CAD build for the part. Positions are in the model's coordinates, mm. A direction names the side the tool comes from. Round coordinates to 2 decimals unless told otherwise and drop trailing zeros. Loops run counter-clockwise (first coordinate to the right, second up) from the corner with the lowest first, then second, coordinate; pieces in that order, holes last.
```python
from build123d import *

# Parameters (mm, degrees)
F0_R     = 13.97
F1_DEPTH = 15.875
F2_R     = 5.08
F3_SIZE2 = 1.27
F3_SIZE  = 1.27
F4_R     = 3.683
F5_DEPTH = 1.778
F6_R     = 1.905
F7_DEPTH = 7.621


with BuildPart() as f1:
    # F0 (on Top) → F1 (new body, symmetric)
    with BuildSketch(Plane.XY):
        with BuildLine():
            Line((3.81, 38.1), (-3.81, 38.1))
            Line((-3.81, 38.1), (-3.81, 23.11151))
            Line((-3.81, 23.11151), (-19.05, 12.95151))
            ThreePointArc((-19.05, 12.95151), (-52.07, 0), (-19.05, -12.95151))
            Line((-19.05, -12.95151), (-3.81, -23.11151))
            Line((-3.81, -23.11151), (-3.81, -38.1))
            Line((-3.81, -38.1), (3.81, -38.1))
            Line((3.81, -38.1), (3.81, 38.1))
        make_face()
        with Locations((-33.02, 0)):
            Circle(F0_R, mode=Mode.SUBTRACT)
    extrude(amount=F1_DEPTH, both=True)

    # F2
    f2_edges = [f1.edges().sort_by_distance(p)[0] for p in [
        (-19.05, -12.95151, 0),
        (-3.81, -23.11151, 0),
        (-3.81, 23.11151, 0),
        (-19.05, 12.95151, 0),
    ]]
    fillet(f2_edges, radius=F2_R)

    # F3
    f3_edges = [f1.edges().sort_by_distance(p)[0] for p in [
        (-46.99, 0, 15.875),
        (-46.99, 0, -15.875),
    ]]
    chamfer(f3_edges, length=F3_SIZE, length2=F3_SIZE2)

    # F4 (on face) → F5 (cut)
    with BuildSketch(Plane(origin=(-3.81, 0, 0), x_dir=(0, -1, 0), z_dir=(-1, 0, 0))):
        with Locations((-31.75, 8.255)):
            Circle(F4_R)
        with Locations((-31.75, -8.255)):
            Circle(F4_R)
        with Locations((31.75, 8.255)):
            Circle(F4_R)
        with Locations((31.75, -8.255)):
            Circle(F4_R)
    extrude(amount=-F5_DEPTH, mode=Mode.SUBTRACT)

    # F6 (on face) → F7 (cut, through all)
    with BuildSketch(Plane(origin=(-3.81, 0, 0), x_dir=(0, -1, 0), z_dir=(-1, 0, 0))):
        with Locations((31.75, 8.255)):
            Circle(F6_R)
        with Locations((-31.75, 8.255)):
            Circle(F6_R)
        with Locations((31.75, -8.255)):
            Circle(F6_R)
        with Locations((-31.75, -8.255)):
            Circle(F6_R)
    extrude(amount=-F7_DEPTH, mode=Mode.SUBTRACT)


solid = f1.part
```
Item 1: Cut at A-A, the plane y = 31.75. Give the cut face in (x, z) (3 decimals), plus the area to 3 significant figures.
Answers follow:
outline: (-3.81, -15.875) - (3.81, -15.875) - (3.81, -10.16) - (-2.032, -10.16) - (-2.032, -11.938) - (-3.81, -11.938) - close; (-3.81, -4.572) - (-2.032, -4.572) - (-2.032, -6.35) - (3.81, -6.35) - (3.81, 6.35) - (-2.032, 6.35) - (-2.032, 4.572) - (-3.81, 4.572) - close; (-3.81, 11.938) - (-2.032, 11.938) - (-2.032, 10.16) - (3.81, 10.16) - (3.81, 15.875) - (-3.81, 15.875) - close
area: 171 mm2
Item 2: Cut at C-C, the plane x = -33.02. Give the cut face in (y, z) (3 decimals), plus the area to 3 significant figures.
Answers follow:
outline: (-19.05, -15.875) - (-15.24, -15.875) - (-13.97, -14.605) - (-13.97, 14.605) - (-15.24, 15.875) - (-19.05, 15.875) - close; (13.97, -14.605) - (15.24, -15.875) - (19.05, -15.875) - (19.05, 15.875) - (15.24, 15.875) - (13.97, 14.605) - close
area: 319 mm2
Item 3: Cut at D-D, the plane y = 0. Give the cut face in (x, z) (3 decimals), plus the area to 3 significant figures.
Answers follow:
outline: (-52.07, -15.875) - (-48.26, -15.875) - (-46.99, -14.605) - (-46.99, 14.605) - (-48.26, 15.875) - (-52.07, 15.875) - close; (-19.05, -14.605) - (-17.78, -15.875) - (3.81, -15.875) - (3.81, 15.875) - (-17.78, 15.875) - (-19.05, 14.605) - close
area: 884 mm2
Item 4: Cut at B-B, the plane z = 0.5. Give the cut face in (x, y), plus the area to 3 significant figures.
Answers follow:
outline: (-21.64, -15.28) arc R5.08 cw to (-15.79, -15.13) - (-6.07, -21.6) arc R5.08 cw to (-3.81, -25.83) - (-3.81, -38.1) - (3.81, -38.1) - (3.81, 38.1) - (-3.81, 38.1) - (-3.81, 25.83) arc R5.08 cw to (-6.07, 21.6) - (-15.79, 15.13) arc R5.08 cw to (-21.64, 15.28) arc R19.05 ccw (long way) to start; hole circle Ø27.94 at (-33.02, 0)
area: 1,570 mm2
Item 5: 3-axis set-ups, long thin cutter, end or side, ignore diameter. For faces 1 (the flat face through (-12, 0, 15.875)), 2 (the cylindrical face through (-2.933, 34.465, 10.744)), 3 (the flat face through (-3.81, -32, 0)): which of +Z, -Z, +X, -X, +Y, -Y reach the whole face in a straight line?
Answers follow:
face 1: +Z, +X, -X, +Y, -Y
face 2: -X
face 3: +Z, -Z, -X, -Y
Item 6: Two-plate mould, pull along X, no slides. Class faces 4 (the flat face through (-3.81, 32, 0)), 5 (the cylindrical face through (0.848, -29.847, -8.171)), 6 (the cylindrical face through (-52.06, 0.59, 0.22)): released by +X, released by -X, zero draft, split by the parting line, or undercut.
Answers follow:
face 4: released by -X
face 5: zero draft
face 6: undercut
Item 7: Probe line 1 (Z direction, x = -2.65, y = 31.75) (3 decimals); line 2 (Z direction, x = 1, y = 31) (3 decimals); line 3 (Y direction, x = -39, z = -7). List the from-to ranges inside material, lowest first.
Answers follow:
line 1: z = -15.875 to -11.938, -4.572 to 4.572, 11.938 to 15.875
line 2: z = -15.875 to -10.006, -6.504 to 6.504, 10.006 to 15.875
line 3: y = -18.09 to -12.63, 12.63 to 18.09
Item 8: Flat gauge pins, fed straight in: P1, Ø13.5, axis at y = 35, z = 7.5, coming from the -X side; P2, Ø5, axis at x = -22.5, y = 8.5, coming from the -Z side (3 decimals); P3, Ø12, axis at x = -39, z = 10.5, coming from the +Y side; P4, Ø3, axis at x = -34, z = 4, coming from the -Y side. Where does each tip first touch, or does it go through?
Answers follow:
P1: stops at x = -3.81
P2: stops at z = -15.875
P3: stops at y = 19.05
P4: stops at y = -19.05
